from build123d import *

# Parameters (mm, degrees)
SKETCH3_W                                        = 226.06
SKETCH3_H                                        = 149.86
EXTRUDE2_DEPTH                                   = 12.7
F_1_4_20_TAPPED_HOLE1_D                          = 5.1054
CBORE_FOR_5_8_SOCKET_HEAD_CAP_SCREW1_D           = 18.6436
CBORE_FOR_5_8_SOCKET_HEAD_CAP_SCREW1_CBORE_D     = 38.1
CBORE_FOR_5_8_SOCKET_HEAD_CAP_SCREW1_CBORE_DEPTH = 2.54
F_10_32_TAPPED_HOLE1_D                           = 4.0386
CHAMFER1_SIZE                                    = 12.7
SKETCH20_R                                       = 19.05
CUT_EXTRUDE5_DEPTH                               = 1.524


with BuildPart() as part:
    # Sketch3 → Extrude2 (new body)
    with BuildSketch(Plane.XY):
        with Locations((113.03, -74.93)):
            Rectangle(SKETCH3_W, SKETCH3_H)
    extrude(amount=EXTRUDE2_DEPTH)

    # 1/4-20 Tapped Hole1 (through all)
    with Locations(Plane(origin=(0, 0, 0), x_dir=(-1, 0, 0), z_dir=(0, 0, -1))):
        with Locations((-195.58, -20.955), (-195.58, -128.905), (-30.48, -43.18), (-30.48, -106.68)):
            Hole(F_1_4_20_TAPPED_HOLE1_D / 2)

    # CBORE for 5/8 Socket Head Cap Screw1 (through all)
    with Locations(Plane(origin=(163.83, -24.13, 0), x_dir=(-1, 0, 0), z_dir=(0, 0, -1))):
        with Locations((0, 0), (101.6, 0), (101.6, -101.6), (0, -101.6)):
            CounterBoreHole(CBORE_FOR_5_8_SOCKET_HEAD_CAP_SCREW1_D / 2, CBORE_FOR_5_8_SOCKET_HEAD_CAP_SCREW1_CBORE_D / 2, CBORE_FOR_5_8_SOCKET_HEAD_CAP_SCREW1_CBORE_DEPTH)

    # #10-32 Tapped Hole1 (through all)
    with Locations(Plane(origin=(0, 0, 0), x_dir=(-1, 0, 0), z_dir=(0, 0, -1))):
        with Locations((-113.03, -13.0048), (-125.73, -136.8552), (-100.33, -136.8552)):
            Hole(F_10_32_TAPPED_HOLE1_D / 2)

    # Chamfer1
    chamfer1_edges = [part.edges().sort_by_distance(p)[0] for p in [
        (0, 0, 6.35),
        (226.06, 0, 6.35),
        (226.06, -149.86, 6.35),
        (0, -149.86, 6.35),
    ]]
    chamfer(chamfer1_edges, length=CHAMFER1_SIZE)

    # Sketch20 → Cut-Extrude5 (cut)
    with BuildSketch(Plane.XY.offset(12.7)):
        with Locations(Location((163.83, -125.73, 0), (0, 0, 180))):  # turned: the seam where the file's is
            Circle(SKETCH20_R)
        with Locations(Location((62.23, -125.73, 0), (0, 0, 180))):  # turned: the seam where the file's is
            Circle(SKETCH20_R)
        with Locations(Location((163.83, -24.13, 0), (0, 0, 180))):  # turned: the seam where the file's is
            Circle(SKETCH20_R)
        with Locations(Location((62.23, -24.13, 0), (0, 0, 180))):  # turned: the seam where the file's is
            Circle(SKETCH20_R)
    extrude(amount=-CUT_EXTRUDE5_DEPTH, mode=Mode.SUBTRACT)


solid = part.part
Part model, mm, in its own coordinate system. A direction names the side the tool comes from. Round coordinates to 2 decimals unless told otherwise and drop trailing zeros. Loops run counter-clockwise (first coordinate to the right, second up) from the corner with the lowest first, then second, coordinate; pieces in that order, holes last. Notation, with made-up numbers: (82.25, -8) - (132.25, -8) arc R28 ccw to (132.25, 13) - close; hole circle Ø11 at (23.5, 2.25). An arc over 180 degrees is marked (long way). Answer as a JSON object with one key per item and string values.
Item 1: Tool access for faces 1 (the face through (76.271, -11.255, 1.252)), 2 (the face through (111, -74, 0)), 3 (the face through (145.66, -131.45, 11.95)): list every direction of +Z, -Z, +X, -X, +Y, -Y with a clear straight run to the whole face (end or side of a thin tool).
Output:
{"face 1": "-Z", "face 2": "-Z, +X, -X, +Y, -Y", "face 3": "+Z"}
Item 2: Pin check, flat tips, straight feed: pin 1 (23 mm diameter, centred on x = 163.83, y = -125.73, fed in from +Z); pin 2 (4.5 mm diameter, centred on x = 30.48, y = -43.18, fed in from +Z); pin 3 (23 mm diameter, centred on x = 163.83, y = -24.13, fed in from -Z). Stop position of each tip, or through.
Output:
{"pin 1": "z = 11.18", "pin 2": "through", "pin 3": "z = 2.54"}
Item 3: Pull direction X, two halves, no side cores. Call faces 4 (the face through (112, 0, 6)), 5 (the face through (6.44, -143.6, 6.26)), 6 (the face through (172.72, -21.33, 6.92)): pulls with the +X half, pulls with the -X half, needs draft (parallel to the pull), parting line crosses it, or undercut.
Output:
{"face 4": "needs draft", "face 5": "pulls with the -X half", "face 6": "undercut"}
Item 4: Wall check: L1, parallel to Y at x = 163.83, z = 7.5; L2, parallel to Y at x = 195.5, z = 7.25; L3, parallel to X at y = -125.73, z = 12.45. Give the ranges that are in metal, low to high.
Output:
{"L1": "-149.86 to -135.05, -116.41 to -33.45, -14.81 to 0", "L2": "-149.86 to -131.46, -126.35 to -23.51, -18.4 to 0", "L3": "0 to 43.18, 81.28 to 144.78, 182.88 to 226.06"}
Item 5: Band-saw the part on A-A on x = 30.48. List the corners of the cut face in (y, z), plus the area to 3 significant figures.
Output:
{"outline": "(-149.86, 0) - (-109.23, 0) - (-109.23, 12.7) - (-149.86, 12.7) - close; (-104.13, 0) - (-45.73, 0) - (-45.73, 12.7) - (-104.13, 12.7) - close; (-40.63, 0) - (0, 0) - (0, 12.7) - (-40.63, 12.7) - close", "area": "1,770 mm2"}
Item 6: Band-saw the part on B-B on z = 8.75. State how many separate pieces and enclosed holes the cut face has, plus the area to 3 significant figures.
Output:
{"separate pieces": "1", "enclosed holes": "11", "area": "32,300 mm2"}
